```python
from build123d import *

# Parameters (mm, degrees)
F0_W     = 128.2316669822
F0_H     = 97.8200212121
F1_DEPTH = 116.2282433361
F2_R     = 38.1
F3_DEPTH = 25.4
F4_R     = 5.08


with BuildPart() as f1:
    # F0 (on Top) → F1 (new body)
    with BuildSketch(Plane.XY):
        with Locations((7.463093847, 4.6752728522)):
            Rectangle(F0_W, F0_H)
    extrude(amount=F1_DEPTH)

    # F2 (on face) → F3 (cut)
    with BuildSketch(Plane.XZ.offset(44.2347377539)):
        with Locations((13.5555826128, 47.6286895573)):
            Circle(F2_R)
    extrude(amount=-F3_DEPTH, mode=Mode.SUBTRACT)

    # F4
    f4_edges = [f1.edges().sort_by_distance(p)[0] for p in [
        (71.578927, -44.234738, 58.114122),
        (7.463094, -44.234738, 116.228243),
        (-24.544417, -44.234738, 47.62869),
    ]]
    fillet(f4_edges, radius=F4_R)


solid = f1.part
```
Input: part model. Units: mm. Frame: model coordinates. A direction names the side the tool comes from. Coordinates: 2 decimals unless noted, no trailing zeros. Loops run counter-clockwise (first coordinate to the right, second up) from the corner with the lowest first, then second, coordinate; pieces in that order, holes last.
Q1. Set-up query: faces 1 (the cylindrical face through (8.596, -29.137, 85.404)), 2 (the flat face through (71.579, 7, 57)). Return all of +Z, -Z, +X, -X, +Y, -Y with unobstructed straight access to the full face (end or side cutting, diameter ignored); none if empty.
Results are:
face 1: -Y
face 2: +Z, -Z, +X, +Y, -Y
Q2. Line query: line 1 along Y through (x, z) = (12.5, 29.5); line 2 along X through (y, z) = (-27, 22); line 3 along Y through (x, z) = (-15.5, 76). Output: solid intervals per line, ascending.
Results are:
line 1: y = -18.83 to 53.59
line 2: x = -56.65 to -14.64, 41.75 to 71.58
line 3: y = -43.54 to 53.59
Q3. Contact query for a flat-ended pin moving along its axis: pin 1 (5 mm diameter, centred on x = -8.5, z = 49.5, fed in from -Y). Output: stop coordinate, or through.
Results are:
pin 1: stops at y = -18.83
Q4. Mould query, pull axis Z, two halves, no side actions, for faces 3 (the flat face through (13, -18.835, 48)), 4 (the flat face through (7, 5, 0)), 5 (the cylindrical face through (70.05, -42.79, 58.93)). Classes: +Z half, -Z half, draft (parallel to the pull), parting line (faces both ways), or undercut.
Results are:
face 3: undercut
face 4: -Z half
face 5: draft
Q5. Section A-A, the plane y = -32.5. Return the cut outline in (x, z).
Results are:
outline: (-56.65, 0) - (71.58, 0) - (71.58, 116.23) - (-56.65, 116.23) - close; hole circle Ø76.2 at (13.56, 47.63)
